Check sheet for the drawn part. Datum: minimum x, y, z corner. Units: mm. A direction names the side the tool comes from. Round coordinates to 2 decimals unless told otherwise and drop trailing zeros. Loops run counter-clockwise (first coordinate to the right, second up) from the corner with the lowest first, then second, coordinate; pieces in that order, holes last. Notation, with made-up numbers: (-30, -40) -> (-17, -40) arc R12 cw to (-17, -31) -> close; hole circle Ø7 at (72.25, -12). An arc over 180 degrees is marked (long way). Return JSON: item names as keys, results as strings.
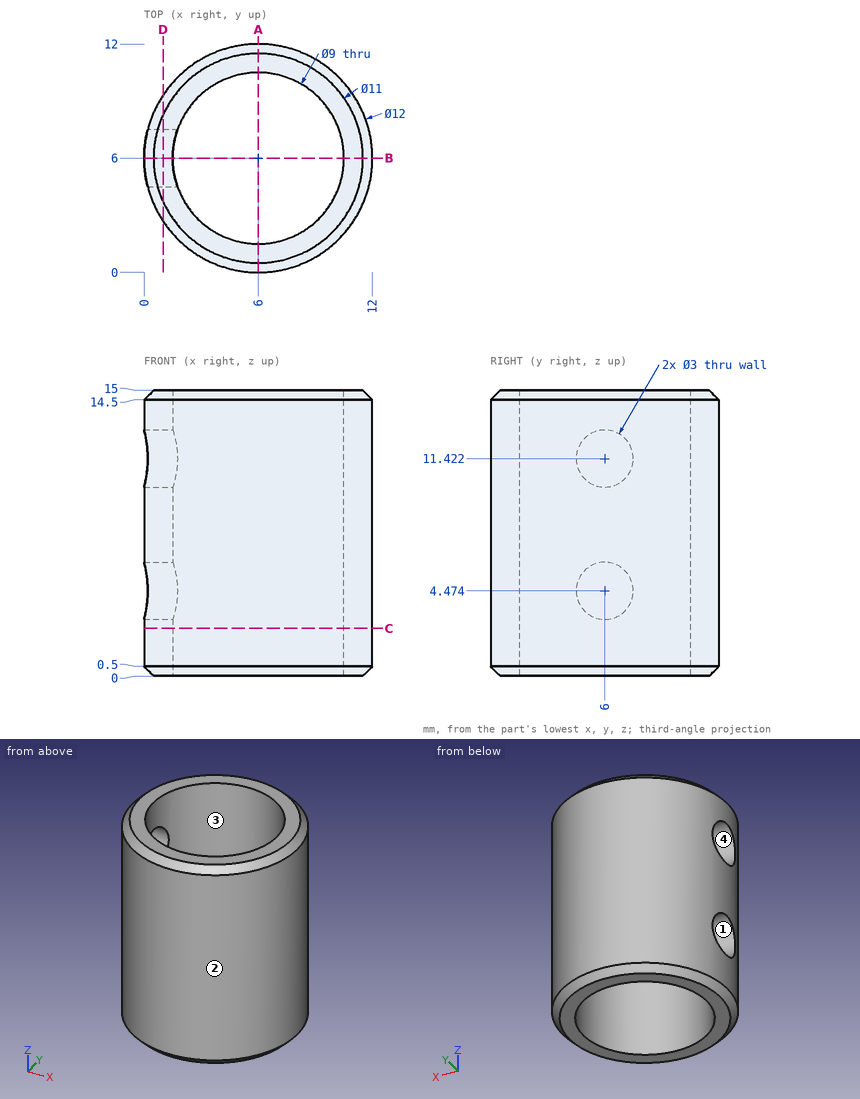
Q1. Draft check along Y on the marked faces 1 and 2. Enter one of: released by +Y, released by -Y, zero draft, split by the parting line, or undercut.
Results list:
{"face 1": "undercut", "face 2": "split by the parting line"}
Q2. Section check B-B (y = 6). Record the boundary of the cut face in (x, z), then the cut area to 3 significant figures.
Results list:
{"outline": "(0, 0.5) -> (0.5, 0) -> (1.5, 0) -> (1.5, 2.97) -> (0, 2.97) -> close; (0, 5.97) -> (1.5, 5.97) -> (1.5, 9.92) -> (0, 9.92) -> close; (0, 12.92) -> (1.5, 12.92) -> (1.5, 15) -> (0.5, 15) -> (0, 14.5) -> close; (10.5, 0) -> (11.5, 0) -> (12, 0.5) -> (12, 14.5) -> (11.5, 15) -> (10.5, 15) -> close", "area": "35.5 mm^2"}
Q3. Section check D-D (x = 1). Count the separate pieces of the cut face and the enclosed holes in it.
Results list:
{"separate pieces": "1", "enclosed holes": "2"}
Q4. Section check C-C (z = 2.5). Record the boundary of the cut face in (x, y).
Results list:
{"outline": "circle Ø12 at (6, 6); hole circle Ø9 at (6, 6)"}
Q5. Section check A-A (x = 6). Record the boundary of the cut face in (y, z), then the cut area to 3 significant figures.
Results list:
{"outline": "(0, 0.5) -> (0.5, 0) -> (1.5, 0) -> (1.5, 15) -> (0.5, 15) -> (0, 14.5) -> close; (10.5, 0) -> (11.5, 0) -> (12, 0.5) -> (12, 14.5) -> (11.5, 15) -> (10.5, 15) -> close", "area": "44.5 mm^2"}
Q6. Go/stop test with flat-tipped pins: pin 1 (4 mm diameter, centred on y = 10, z = 2.5, fed in from +X); pin 2 (2 mm diameter, centred on x = 2, z = 9.5, fed in from -Y); pin 3 (3 mm diameter, centred on y = 3, z = 5.5, fed in from +X). Record where each tip stops, or that it passes through.
Results list:
{"pin 1": "x = 11.66", "pin 2": "y = 0.8", "pin 3": "x = 11.81"}
Q7. Tool access check on the marked faces 3 and 4. Record the directions out of +Z, -Z, +X, -X, +Y, -Y that give a thin tool (end or side, any length) a straight path to the whole face; none if there is none.
Results list:
{"face 3": "+Z, -Z", "face 4": "-X"}
Q8. Material ranges on line 1 (Y direction, x = 6, z = 4.5); line 2 (X direction, y = 4, z = 5); line 3 (Y direction, x = 9.25, z = 2.75) (1 decimal), recorded low to high.
Results list:
{"line 1": "0 to 1.5, 10.5 to 12", "line 2": "0.34 to 1.97, 10.03 to 11.66", "line 3": "1 to 2.9, 9.1 to 11"}
